Build history of the part. All positions in model axes, mm. Face numbers are marked on the shaded views. A direction names the side the tool comes from. Round coordinates to 2 decimals unless told otherwise and drop trailing zeros. Write each loop counter-clockwise with the first axis right and the second up, starting at its lowest first coordinate (ties: lowest second). Pieces come first, ordered by that corner, then holes. Notation, with made-up numbers: (18.25, -36) -> (25.25, -36) arc R26 cw to (25.25, -19) -> close; hole circle Ø4 at (40, -25.5). An arc over 180 degrees is marked (long way). Answer in a Markdown table with one row per item. Add a question column.
from build123d import *

# Parameters (mm, degrees)
F0_R     = 25
F0_R_2   = 17.55
F1_DEPTH = 65
F2_R     = 6
F3_DEPTH = 65.001
F4_R     = 17.55
F5_DEPTH = 27


with BuildPart() as f1:
    # F0 (on Top) → F1 (new body)
    with BuildSketch(Plane.XY):
        Circle(F0_R)
        Circle(F0_R_2, mode=Mode.SUBTRACT)
        Circle(F0_R_2)
    extrude(amount=F1_DEPTH)

    # F2 (on face) → F3 (cut, through all)
    with BuildSketch(Plane(origin=(0, 0, 0), x_dir=(1, 0, 0), z_dir=(0, 0, -1))):
        Circle(F2_R)
    extrude(amount=-F3_DEPTH, mode=Mode.SUBTRACT)

    # F4 (on face) → F5 (cut)
    with BuildSketch(Plane(origin=(0, 0, 0), x_dir=(1, 0, 0), z_dir=(0, 0, -1))):
        Circle(F4_R)
    extrude(amount=-F5_DEPTH, mode=Mode.SUBTRACT)


solid = f1.part
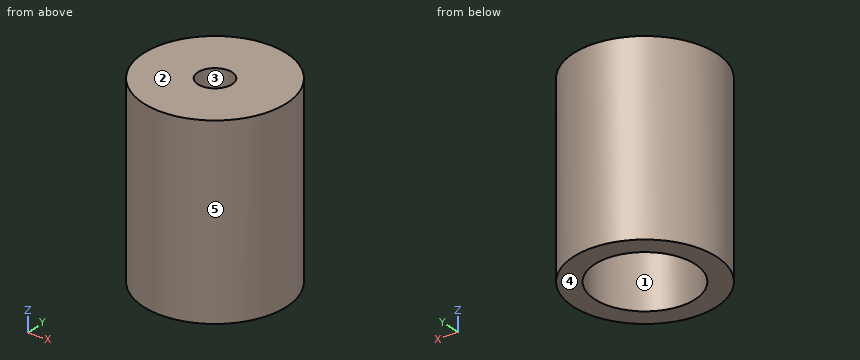
(1) Saw through at A-A (y = 0). List the corners of the cut face in (x, z), plus the area to 3 significant figures.
(2) Saw through at D-D (z = 58.5). List the corners of the cut face in (x, y).
(3) Probe line 1 along Y through (x, z) = (0, 14); line 2 along Y through (x, z) = (0, 50); line 3 along Z through (x, y) = (-16, 1). List the from-to ranges inside material, lowest first.
(4) Saw through at C-C (y = -13.5). List the corners of the cut face in (x, z), plus the area to 3 significant figures.
(5) Which spindle directions (+Z, -Z, +X, -X, +Y, -Y) get a long thin tool onto all of the face, cutting with end or side? Do the marked faces 1 and 2. Say none if no direction does.
(6) Drop flat-ended pins along their axis: P1, Ø6, axis at x = 16.5, z = 47, coming from the +Y side; P2, Ø12, axis at x = -8.5, z = 45.5, coming from the +Y side; P3, Ø12, axis at x = 1.5, z = 50.5, coming from the +Y side. Give the stop position or say it passes through.
(7) Mould opens along X. For the marked faces 3, 4 and 5 say: pulls with the +X half, pulls with the -X half, needs draft (parallel to the pull), parting line crosses it, or undercut.
Answer sheet:
| question | item | result |
|---|---|---|
| 1 | outline | (-25, 0) -> (-17.55, 0) -> (-17.55, 27) -> (-6, 27) -> (-6, 65) -> (-25, 65) -> close; (6, 27) -> (17.55, 27) -> (17.55, 0) -> (25, 0) -> (25, 65) -> (6, 65) -> close |
| 1 | area | 1,850 mm² |
| 2 | outline | circle Ø50 at (0, 0); hole circle Ø12 at (0, 0) |
| 3 | line 1 | y = -25 to -17.55, 17.55 to 25 |
| 3 | line 2 | y = -25 to -6, 6 to 25 |
| 3 | line 3 | z = 27 to 65 |
| 4 | outline | (-21.04, 0) -> (-11.21, 0) -> (-11.21, 27) -> (11.21, 27) -> (11.21, 0) -> (21.04, 0) -> (21.04, 65) -> (-21.04, 65) -> close |
| 4 | area | 2,130 mm² |
| 5 | face 1 | -Z |
| 5 | face 2 | +Z, +X, -X, +Y, -Y |
| 6 | P1 | stops at y = 21.04 |
| 6 | P2 | stops at y = 24.87 |
| 6 | P3 | stops at y = 25 |
| 7 | face 3 | undercut |
| 7 | face 4 | needs draft |
| 7 | face 5 | parting line crosses it |
